```python
from build123d import *

# Parameters (mm, degrees)
SKETCH2_R           = 1.55
BOSS_EXTRUDE1_DEPTH = 1.5
SKETCH3_R           = 10.5
BOSS_EXTRUDE2_DEPTH = 3
SKETCH4_R           = 5
BOSS_EXTRUDE3_DEPTH = 5
SKETCH5_R           = 2.5
CUT_EXTRUDE1_DEPTH  = 28.207535721
CHAMFER1_SIZE       = 0.5


with BuildPart() as part:
    # Sketch2 → Boss-Extrude1 (new body)
    with BuildSketch(Plane.XY):
        with BuildLine():
            Line((-8.485281374, 17), (8.485281374, 17))
            ThreePointArc((8.485281374, 17), (19, 0), (8.485281374, -17))
            Line((8.485281374, -17), (-8.485281374, -17))
            ThreePointArc((-8.485281374, -17), (-19, 0), (-8.485281374, 17))
        make_face()
        with Locations((-16, 0)):
            Circle(SKETCH2_R, mode=Mode.SUBTRACT)
        with Locations((-8, 13.856406461)):
            Circle(SKETCH2_R, mode=Mode.SUBTRACT)
        with Locations((8, 13.856406461)):
            Circle(SKETCH2_R, mode=Mode.SUBTRACT)
        with Locations((16, 0)):
            Circle(SKETCH2_R, mode=Mode.SUBTRACT)
        with Locations((8, -13.856406461)):
            Circle(SKETCH2_R, mode=Mode.SUBTRACT)
        with Locations((-8, -13.856406461)):
            Circle(SKETCH2_R, mode=Mode.SUBTRACT)
    extrude(amount=BOSS_EXTRUDE1_DEPTH)

    # Sketch3 → Boss-Extrude2 (add)
    with BuildSketch(Plane.XY.offset(1.5)):
        Circle(SKETCH3_R)
    extrude(amount=BOSS_EXTRUDE2_DEPTH)

    # Sketch4 → Boss-Extrude3 (add)
    with BuildSketch(Plane(origin=(0, 0, 0), x_dir=(-1, 0, 0), z_dir=(0, 0, -1))):
        Circle(SKETCH4_R)
    extrude(amount=BOSS_EXTRUDE3_DEPTH)

    # Sketch5 → Cut-Extrude1 (cut, through all)
    with BuildSketch(Plane.XY.offset(4.5)):
        Circle(SKETCH5_R)
    extrude(amount=-CUT_EXTRUDE1_DEPTH, mode=Mode.SUBTRACT)

    # Chamfer1
    chamfer1_edges = [part.edges().sort_by_distance(p)[0] for p in [
        (-19, 0, 1.5),
        (-10.5, 0, 4.5),
        (5, 0, -5),
        (19, 0, 1.5),
        (-2.5, 0, -5),
        (-2.5, 0, 4.5),
        (-19, 0, 0),
        (19, 0, 0),
    ]]
    chamfer(chamfer1_edges, length=CHAMFER1_SIZE)


solid = part.part
```
Verification items for the finished model (mm, model axes). A direction names the side the tool comes from. Give positions to 0.01 mm unless a question says otherwise; leave off trailing zeros. Order: outer loops, then holes, each group sorted by start corner. A loop starts at its lowest first (then second) coordinate and runs counter-clockwise, first axis right, second up. Notation, with made-up numbers: (18, 88.25) -> (77, 88.25) arc R11 ccw to (77, 105.25) -> close; hole circle Ø5 at (6.5, -14.75). An arc over 180 degrees is marked (long way). One line per item, written item: value.
(1) Scan lines: line 1 along Y through (x, z) = (8, 0.7); line 2 along Y through (x, z) = (0, 0.5); line 3 along X through (y, z) = (-1, 0.75). Record each from-to range of solid material in increasing order. Write a range as [from, to].
Final values:
line 1: [-17, -15.41], [-12.31, 12.31], [15.41, 17]
line 2: [-17, -2.5], [2.5, 17]
line 3: [-18.97, -17.18], [-14.82, -2.29], [2.29, 14.82], [17.18, 18.97]
(2) Sectioned sample at A-A on x = 0. Record the cut outline in (y, z).
Final values:
outline: (-17, 0) -> (-5, 0) -> (-5, -4.5) -> (-4.5, -5) -> (-3, -5) -> (-2.5, -4.5) -> (-2.5, 4) -> (-3, 4.5) -> (-10, 4.5) -> (-10.5, 4) -> (-10.5, 1.5) -> (-17, 1.5) -> close; (2.5, -4.5) -> (3, -5) -> (4.5, -5) -> (5, -4.5) -> (5, 0) -> (17, 0) -> (17, 1.5) -> (10.5, 1.5) -> (10.5, 4) -> (10, 4.5) -> (3, 4.5) -> (2.5, 4) -> close
(3) Draft check along Y on faces 4 (the face through (-17.55, 0.07, 0.74)), 5 (the face through (2.1, 2.4, 4.5)), 6 (the face through (18.633, 0.304, 1.365)). Enter one of: pulls with the +Y half, pulls with the -Y half, needs draft (parallel to the pull), parting line crosses it, or undercut.
Final values:
face 4: undercut
face 5: needs draft
face 6: parting line crosses it
(4) Sectioned sample at C-C on z = 3. Record the cut outline in (x, y), then the cut area to 3 significant figures.
Final values:
outline: circle Ø21 at (0, 0); hole circle Ø5 at (0, 0)
area: 327 mm^2
(5) Gauge pin test, flat ends, axial feed: pin 1 (5 mm diameter, centred on x = -16, y = 0, fed in from -Z); pin 2 (5 mm diameter, centred on x = 16, y = 0, fed in from +Z). Record the tip position at first contact, or that the pin passes through.
Final values:
pin 1: z = 0
pin 2: z = 1.5
(6) Sectioned sample at B-B on y = 0. Count the separate pieces of the cut face and the enclosed holes in it, then the cut area to 3 significant figures.
Final values:
separate pieces: 4
enclosed holes: 0
area: 112 mm^2
(7) Tool access check on faces 1 (the face through (10, 3.2, 2.7)), 2 (the face through (1.08, -4.88, -2.22)), 3 (the face through (18.633, 0.304, 0.135)). Record the directions out of +Z, -Z, +X, -X, +Y, -Y that give a thin tool (end or side, any length) a straight path to the whole face; none if there is none.
Final values:
face 1: +Z
face 2: -Z
face 3: -Z, +X
